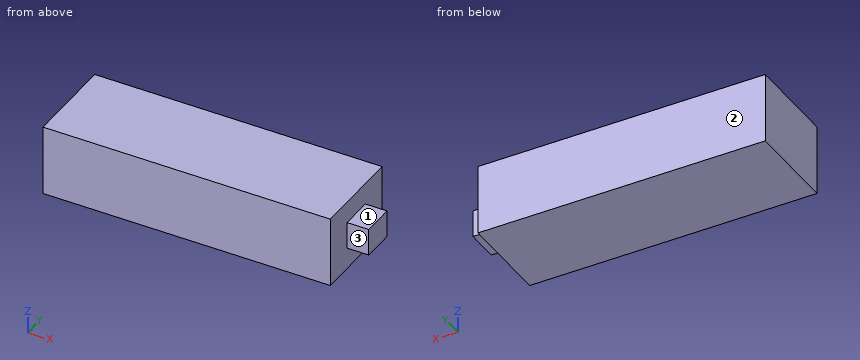
from build123d import *

# Parameters (mm, degrees)
SKETCH1_W       = 106
SKETCH1_H       = 34
PACK_2_DEPTH    = 26
SKETCH2_W       = 8
SKETCH2_H       = 12
LEAD_EXIT_DEPTH = 10


with BuildPart() as part:
    # Sketch1 → Pack 2 (new body)
    with BuildSketch(Plane.XY):
        Rectangle(SKETCH1_W, SKETCH1_H)
    extrude(amount=PACK_2_DEPTH)

    # Sketch2 → Lead_exit (add)
    with BuildSketch(Plane.XY.offset(8)):
        with Locations((57, 0)):
            Rectangle(SKETCH2_W, SKETCH2_H)
    extrude(amount=LEAD_EXIT_DEPTH)


solid = part.part
The listing builds one solid part. Answer for the finished solid, in the listing's coordinates (mm). Face numbers are marked on the shaded views. A direction names the side the tool comes from. Coordinates: 2 decimals unless noted, no trailing zeros. Write each loop counter-clockwise with the first axis right and the second up, starting at its lowest first coordinate (ties: lowest second). Pieces come first, ordered by that corner, then holes. Notation, with made-up numbers: (0.25, 27.5) - (13.25, 27.5) arc R30 cw to (13.25, 60.5) - close; hole circle Ø8 at (-31.75, 79.25). An arc over 180 degrees is marked (long way). Return JSON: item names as keys, results as strings.
1. Which of the six approach directions +Z, -Z, +X, -X, +Y, -Y give full straight-line access (tool end or side, diameter ignored) to the marked faces 1, 2 and 3?
Final values:
{"face 1": "+Z, +X, +Y, -Y", "face 2": "+Z, -Z, +X, -X, +Y", "face 3": "+Z, -Z, +X, -Y"}
2. The part is cut by section A-A on y = -2. Determine the outline of the cut face in (x, z).
Final values:
{"outline": "(-53, 0) - (53, 0) - (53, 8) - (61, 8) - (61, 18) - (53, 18) - (53, 26) - (-53, 26) - close"}
3. Each of these flat-tipped pins is pushed along its axis until it touches: pin 1 Ø4 at (x, y) = (55.5, -3) entering from +Z; pin 2 Ø10 at (y, z) = (13.5, 14.5) entering from +X; pin 3 Ø2.5 at (x, z) = (58.5, 13.5) entering from +Y. Where does it stop, or does it pass through?
Final values:
{"pin 1": "z = 18", "pin 2": "x = 53", "pin 3": "y = 6"}
4. The part is cut by section D-D on z = 1.5. Determine the outline of the cut face in (x, y), then the cut area to 3 significant figures.
Final values:
{"outline": "(-53, -17) - (53, -17) - (53, 17) - (-53, 17) - close", "area": "3,600 mm^2"}
5. The part is cut by section C-C on y = 14. Determine the outline of the cut face in (x, z), then the cut area to 3 significant figures.
Final values:
{"outline": "(-53, 0) - (53, 0) - (53, 26) - (-53, 26) - close", "area": "2,760 mm^2"}
6. The part is cut by section B-B on z = 9.5. Determine the outline of the cut face in (x, y), then the cut area to 3 significant figures.
Final values:
{"outline": "(-53, -17) - (53, -17) - (53, -6) - (61, -6) - (61, 6) - (53, 6) - (53, 17) - (-53, 17) - close", "area": "3,700 mm^2"}
7. Consider line 1 along X through (y, z) = (-0.5, 4). Determine where the line is inside the solid, lowest interval first.
Final values:
{"line 1": "-53 to 53"}
